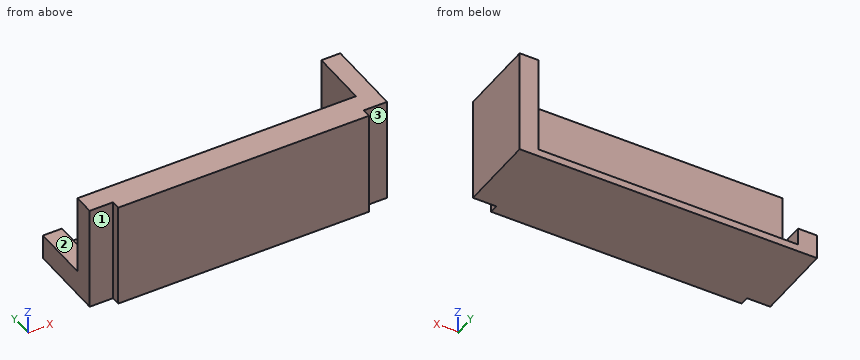
```python
from build123d import *

# Parameters (mm, degrees)
ESQUISSE2_W             = 43
ESQUISSE2_H             = 18
BOSS_EXTRU_1_DEPTH      = 3.5
BOSS_EXTRU_1_DEPTH_BACK = 1.5
ESQUISSE3_W             = 18
ESQUISSE3_H             = 3.5
BOSS_EXTRU_2_DEPTH      = 4
ESQUISSE4_W             = 18
ESQUISSE4_H             = 3.5
BOSS_EXTRU_3_DEPTH      = 4
ESQUISSE5_W             = 51
ESQUISSE5_H             = 1.25
BOSS_EXTRU_4_DEPTH      = 10
ESQUISSE6_W             = 3.25
ESQUISSE6_H             = 16.75
BOSS_EXTRU_5_DEPTH      = 10
ESQUISSE7_W             = 3.25
ESQUISSE7_H             = 3
BOSS_EXTRU_6_DEPTH      = 10


with BuildPart() as part:
    # Esquisse2 → Boss.-Extru.1 (new body, two sides)
    with BuildSketch(Plane(origin=(0, 0, 0), x_dir=(1, 0, 0), z_dir=(0, 1, 0))) as boss_extru_1_sk:
        with Locations((21.5, 9)):
            Rectangle(ESQUISSE2_W, ESQUISSE2_H)
    extrude(amount=BOSS_EXTRU_1_DEPTH)
    extrude(boss_extru_1_sk.sketch, amount=-BOSS_EXTRU_1_DEPTH_BACK)

    # Esquisse3 → Boss.-Extru.2 (add)
    with BuildSketch(Plane(origin=(43, 0, 0), x_dir=(0, 0, -1), z_dir=(1, 0, 0))):
        with Locations((9, 1.75)):
            Rectangle(ESQUISSE3_W, ESQUISSE3_H)
    extrude(amount=BOSS_EXTRU_2_DEPTH)

    # Esquisse4 → Boss.-Extru.3 (add)
    with BuildSketch(Plane.ZY):
        with Locations((-9, 1.75)):
            Rectangle(ESQUISSE4_W, ESQUISSE4_H)
    extrude(amount=BOSS_EXTRU_3_DEPTH)

    # Esquisse5 → Boss.-Extru.4 (add)
    with BuildSketch(Plane(origin=(0, 3.5, 0), x_dir=(1, 0, 0), z_dir=(0, 1, 0))):
        with Locations((21.5, 17.375)):
            Rectangle(ESQUISSE5_W, ESQUISSE5_H)
    extrude(amount=BOSS_EXTRU_4_DEPTH)

    # Esquisse6 → Boss.-Extru.5 (add)
    with BuildSketch(Plane(origin=(0, 3.5, 0), x_dir=(1, 0, 0), z_dir=(0, 1, 0))):
        with Locations((45.375, 8.375)):
            Rectangle(ESQUISSE6_W, ESQUISSE6_H)
    extrude(amount=BOSS_EXTRU_5_DEPTH)

    # Esquisse7 → Boss.-Extru.6 (add)
    with BuildSketch(Plane(origin=(0, 3.5, 0), x_dir=(1, 0, 0), z_dir=(0, 1, 0))):
        with Locations((-2.375, 15.25)):
            Rectangle(ESQUISSE7_W, ESQUISSE7_H)
    extrude(amount=BOSS_EXTRU_6_DEPTH)


solid = part.part
```
Design review of the part built by this model. Coordinates are the model's own, in mm. Face numbers are marked on the shaded views. A direction names the side the tool comes from. Give positions to 0.01 mm unless a question says otherwise; leave off trailing zeros. Loops run counter-clockwise (first coordinate to the right, second up) from the corner with the lowest first, then second, coordinate; pieces in that order, holes last. Notation, with made-up numbers: (37.5, -4.75) -> (90.5, -4.75) arc R21 cw to (90.5, 14.25) -> close; hole circle Ø7 at (-12.75, 9.5). An arc over 180 degrees is marked (long way). Write each question's results on one line, items separated by ' | '.
Q1. Take a section at A-A, the plane y = 12. Write out the cut boundary in (x, z).
Reply:
outline: (-4, -18) -> (47, -18) -> (47, 0) -> (43.75, 0) -> (43.75, -16.75) -> (-0.75, -16.75) -> (-0.75, -13.75) -> (-4, -13.75) -> close
Q2. Wall thickness on L1, parallel to Y at x = 38.5, z = -8; L2, parallel to Z at x = 13, y = 8.5; L3, parallel to Y at x = 44, z = -0.75: over which ranges is each line inside the solid? List them lowest first.
Reply:
L1: y = -1.5 to 3.5 | L2: z = -18 to -16.75 | L3: y = 0 to 13.5
Q3. For pin 1 Ø3 at (x, y) = (17.5, 8) entering from +Z; pin 2 Ø0.8 at (y, z) = (-1, -10) entering from -X; pin 3 Ø1 at (x, y) = (-3, 10) entering from +Z, all flat-tipped, find the tip position at first contact; note any pin that passes through.
Reply:
pin 1: stops at z = -16.75 | pin 2: stops at x = 0 | pin 3: stops at z = -13.75
Q4. Machinability: for the marked faces 1, 2 and 3, which of the approach directions +Z, -Z, +X, -X, +Y, -Y give a long, thin tool a straight path to every point of the face, cutting with its end or side? Answer none if there is none.
Reply:
face 1: +Z, -Z, -X, -Y | face 2: +Z, -X, +Y | face 3: +Z, -Z, +X, -Y
Q5. Take a section at B-B, the plane z = -11. Write out the cut boundary in (x, y), plus the area to 4 significant figures.
Reply:
outline: (-4, 0) -> (0, 0) -> (0, -1.5) -> (43, -1.5) -> (43, 0) -> (47, 0) -> (47, 13.5) -> (43.75, 13.5) -> (43.75, 3.5) -> (-4, 3.5) -> close | area: 275.5 mm²
Q6. Take a section at C-C, the plane x = 10. Write out the cut boundary in (y, z), plus the area to 4 significant figures.
Reply:
outline: (-1.5, -18) -> (13.5, -18) -> (13.5, -16.75) -> (3.5, -16.75) -> (3.5, 0) -> (-1.5, 0) -> close | area: 102.5 mm²
